Build history of the part. All positions in model axes, mm. Face numbers are marked on the shaded views. Round coordinates to 2 decimals unless told otherwise and drop trailing zeros. Loops run counter-clockwise (first coordinate to the right, second up) from the corner with the lowest first, then second, coordinate; pieces in that order, holes last. Notation, with made-up numbers: (37, -26.75) -> (71, -26.75) arc R18 ccw to (71, -7.75) -> close; hole circle Ø4 at (5.25, -8.75). An arc over 180 degrees is marked (long way). Put each result on its own line as item: value. Start each with the question number.
Item 1: Pull direction X, two halves, no side cores. Call the marked faces 1, 2 and 3: +X half, -X half, draft (parallel to the pull), parting line (faces both ways), or undercut.
Item 2: Drill centre lines: probe 1 along Y at (x, z) = (0, 24.6); probe 2 along X at (y, z) = (5.5, 17.75); probe 3 along X at (y, z) = (-8.25, 21.25). Where is each one in solid material? Low to high. Write a range as [from, to].
Item 3: Flat gauge pins, fed straight in: pin 1 Ø6 at (y, z) = (-7.5, 3.5) entering from -X (3 decimals); pin 2 Ø12 at (x, z) = (-5, 20) entering from -Y; pin 3 Ø5 at (x, y) = (5.5, 3.5) entering from -Z; pin 4 Ø1.8 at (x, y) = (0, 0) entering from -Z. Where does each tip first touch, or does it go through?
Item 4: Cut at D-D, the plane y = -8. List the corners of the cut face in (x, z).
Item 5: Cut at C-C, the plane x = -4. List the corners of the cut face in (y, z), plus the area to 3 significant figures.
Item 6: Cut at B-B, the plane z = 21.75. List the corners of the cut face in (x, y).
Item 7: Cut at A-A, the plane y = 0. List the corners of the cut face in (x, z), plus the area to 3 significant figures.
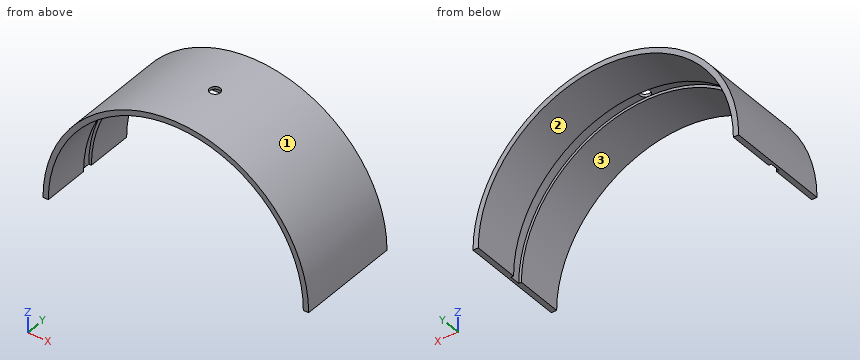
```python
from build123d import *

# Parameters (mm, degrees)
F1_DEPTH = 10
F2_W     = 0.5
F2_H     = 2
F4_R     = 1
F5_DEPTH = 25.001


with BuildPart() as f1:
    # F0 (on Front) → F1 (new body, symmetric)
    with BuildSketch(Plane.XZ):
        with BuildLine():
            Line((24, 0), (25, 0))
            ThreePointArc((25, 0), (0, 25), (-25, 0))
            Line((-25, 0), (-24, 0))
            ThreePointArc((-24, 0), (0, 24), (24, 0))
        make_face()
    extrude(amount=F1_DEPTH, both=True)

    # F2 (on Top) → F3 (revolve, cut)
    with BuildSketch(Plane.XY):
        with Locations((-24.25, 0)):
            Rectangle(F2_W, F2_H)
    revolve(axis=Axis((0, 0, 0), (0, -1, 0)), mode=Mode.SUBTRACT)

    # F4 (on Top) → F5 (cut, through all)
    with BuildSketch(Plane.XY):
        Circle(F4_R)
    extrude(amount=F5_DEPTH, mode=Mode.SUBTRACT)


solid = f1.part
```
Reply:
1. face 1: parting line
1. face 2: undercut
1. face 3: undercut
2. probe 1: y = [-10, -1], [1, 10]
2. probe 2: x = [-17.61, -16.15], [16.15, 17.61]
2. probe 3: x = [-13.17, -11.16], [11.16, 13.17]
3. pin 1: stops at x = -24.995
3. pin 2: stops at y = -10
3. pin 3: stops at z = 22.63
3. pin 4: passes through
4. outline: (-25, 0) -> (-24, 0) arc R24 cw to (24, 0) -> (25, 0) arc R25 ccw to start
5. outline: (-10, 23.66) -> (-1, 23.66) -> (-1, 24.17) -> (1, 24.17) -> (1, 23.66) -> (10, 23.66) -> (10, 24.68) -> (-10, 24.68) -> close
5. area: 19.3 mm^2
6. outline: (-12.33, -10) -> (-10.15, -10) -> (-10.15, -1) -> (-11.28, -1) -> (-11.28, 1) -> (-10.15, 1) -> (-10.15, 10) -> (-12.33, 10) -> close; (10.15, -10) -> (12.33, -10) -> (12.33, 10) -> (10.15, 10) -> (10.15, 1) -> (11.28, 1) -> (11.28, -1) -> (10.15, -1) -> close
7. outline: (-25, 0) -> (-24.5, 0) arc R24.5 cw to (-1, 24.48) -> (-1, 24.98) arc R25 ccw to start; (1, 24.48) arc R24.5 cw to (24.5, 0) -> (25, 0) arc R25 ccw to (1, 24.98) -> close
7. area: 37.9 mm^2
